Check sheet for the modelled part. Datum: model origin and axes. Units: mm. Round coordinates to 2 decimals unless told otherwise and drop trailing zeros. Loops run counter-clockwise (first coordinate to the right, second up) from the corner with the lowest first, then second, coordinate; pieces in that order, holes last. Notation, with made-up numbers: (-23.75, 27) - (12.25, 27) arc R21 cw to (12.25, 65) - close; hole circle Ø6 at (-5.5, 84). An arc over 180 degrees is marked (long way). Answer in a Markdown table with one row per item. Add a question column.
(1) Cross-section at C-C on x = 36. Enter the section's corners in (y, z), then the cut area to 3 significant figures.
(2) Thickness scan on line 1 along Z through (x, y) = (15, 1.5); line 2 along Z through (x, y) = (4.5, 3.9); line 3 along X through (y, z) = (3.35, 45.5). Record the ranges inside material, lowest first.
(3) Cross-section at A-A on x = -15. Enter the section's corners in (y, z).
(4) Cross-section at D-D on z = 15. Count the separate pieces of the cut face and the enclosed holes in it, then the cut area to 3 significant figures.
(5) Gauge pin test, flat ends, axial feed: pin 1 (4.5 mm diameter, centred on x = -47, z = 15, fed in from +Y); pin 2 (2 mm diameter, centred on x = 41, y = 3.5, fed in from +Z); pin 3 (2 mm diameter, centred on x = 42.5, y = 3.5, fed in from -Z); pin 4 (2 mm diameter, centred on x = 43, z = -6, fed in from +Y). Record the tip position at first contact, or that the pin passes through.
from build123d import *

# Parameters (mm, degrees)
BOSS_EXTRUDE3_DEPTH             = 4.5
CUT_EXTRUDE4_DEPTH              = 96.5
CUT_EXTRUDE5_DEPTH              = 32.5
F_4_0MM_PRESS_DOWEL_HOLE3_D     = 3.8
F_4_0MM_PRESS_DOWEL_HOLE3_DEPTH = 57
F_4_0MM_PRESS_DOWEL_HOLE3_TIP   = 4.587005769


with BuildPart() as part:
    # Sketch9 → Boss-Extrude3 (new body)
    with BuildSketch(Plane(origin=(0, 0, 0), x_dir=(1, 0, 0), z_dir=(0, 1, 0))):
        Polygon((19.003020228, -51.996979772), (-18.996979772, -51.996979772), (-51.996979772, -18.996979772), (-51.996979772, 18.996979772), (-18.996979772, 51.996979772), (19.003020228, 51.996979772), (49.493959544, 21.5), (49.493959544, -21.5), align=None)
        Polygon((-41.996979772, -18.996979772), (-41.996979772, 18.996979772), (-18.996979772, 41.996979772), (18.996979772, 41.996979772), (38.993959544, 22), (38.993959544, -22), (18.996979772, -41.996979772), (-18.996979772, -41.996979772), align=None, mode=Mode.SUBTRACT)
    extrude(amount=BOSS_EXTRUDE3_DEPTH)

    # Sketch13 → Cut-Extrude4 (cut)
    with BuildSketch(Plane.XY.offset(51.996979772)):
        Polygon((64.276727826, 15.051195438), (49.5, 0), (43.14121867, 4.5), (43.14121867, 18.660375199), align=None)
    extrude(amount=-CUT_EXTRUDE4_DEPTH, mode=Mode.SUBTRACT)

    # Sketch14 → Cut-Extrude5 (cut)
    with BuildSketch(Plane.ZY.offset(-38.993959544)):
        Polygon((-22, 4.5), (-22, 2.563194296), (22, 2.563194296), (22, 4.5), (18.996979772, 4.5), (-18.996979772, 4.5), align=None)
    extrude(amount=-CUT_EXTRUDE5_DEPTH, mode=Mode.SUBTRACT)

    # Ø4.0mm Press Dowel Hole3
    with Locations(Plane(origin=(0, 4.5, 0), x_dir=(1, 0, 0), z_dir=(0, 1, 0))):
        with Locations((-46.996979772, -15), (-15, 46.996979772), (-46.996979772, 15), (15, 46.996979772), (15, -46.996979772), (-15, -46.996979772)):
            Hole(F_4_0MM_PRESS_DOWEL_HOLE3_D / 2, depth=F_4_0MM_PRESS_DOWEL_HOLE3_DEPTH)
            with Locations((0, 0, -(F_4_0MM_PRESS_DOWEL_HOLE3_DEPTH + F_4_0MM_PRESS_DOWEL_HOLE3_TIP / 2))):  # 45° drill point
                Cone(0, F_4_0MM_PRESS_DOWEL_HOLE3_D / 2, F_4_0MM_PRESS_DOWEL_HOLE3_TIP, mode=Mode.SUBTRACT)


solid = part.part
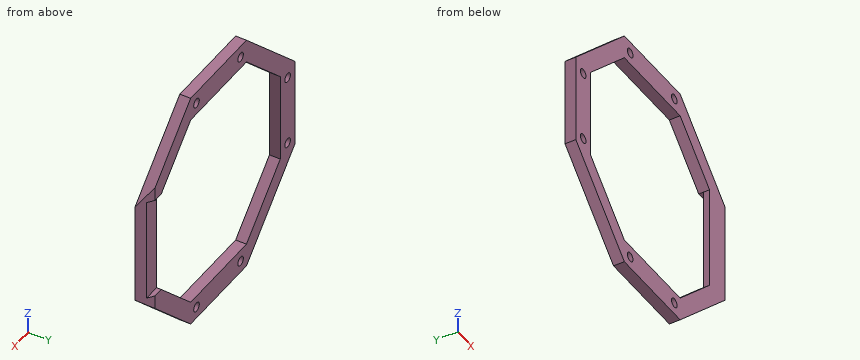
Answers:
| question | item | result |
|---|---|---|
| 1 | outline | (0, -35) - (4.5, -35) - (4.5, -24.99) - (0, -24.99) - close; (0, 24.99) - (4.5, 24.99) - (4.5, 35) - (0, 35) - close |
| 1 | area | 90.0 mm^2 |
| 2 | line 1 | z = -52 to -48.9, -45.1 to -42, 42 to 45.1, 48.9 to 52 |
| 2 | line 2 | z = -52 to -42, 42 to 52 |
| 2 | line 3 | x = -25.49 to -16.17, -13.83 to 13.83, 16.17 to 25.5 |
| 3 | outline | (0, -52) - (4.5, -52) - (4.5, -48.9) - (0, -48.9) - close; (0, -45.1) - (4.5, -45.1) - (4.5, -42) - (0, -42) - close; (0, 42) - (4.5, 42) - (4.5, 45.1) - (0, 45.1) - close; (0, 48.9) - (4.5, 48.9) - (4.5, 52) - (0, 52) - close |
| 4 | separate pieces | 3 |
| 4 | enclosed holes | 0 |
| 4 | area | 50.2 mm^2 |
| 5 | pin 1 | stops at y = 4.5 |
| 5 | pin 2 | stops at z = 31 |
| 5 | pin 3 | stops at z = -29.5 |
| 5 | pin 4 | stops at y = 2.56 |
